Work out the finished part from the listing and answer in its coordinate system (mm). Face numbers are marked on the shaded views. A direction names the side the tool comes from. Coordinates: 2 decimals unless noted, no trailing zeros. Order: outer loops, then holes, each group sorted by start corner. A loop starts at its lowest first (then second) coordinate and runs counter-clockwise, first axis right, second up. Notation, with made-up numbers: M 45,-24.5 L 73,-24.5 A18 ccw 73,5.5 Z; hole C 17.25,10.5 d1. An arc over 180 degrees is marked long. Answer in a Markdown table with one row per item. Add a question column.
Item 1: The part is cut by section A-A (z = 4). Write down the section's boundary in (x, y), then the cut area to 3 significant figures.
Item 2: Which of the six approach directions +Z, -Z, +X, -X, +Y, -Y give full straight-line access (tool end or side, diameter ignored) to the marked faces 4, 5, 6 and 7?
Item 3: Consider line 1 (X direction, y = 8.25, z = -15); line 2 (Y direction, x = -2.5, z = -71); line 3 (Y direction, x = 17, z = -2). Determine where each line is inside the solid, lowest interval first. Write a range as from..to.
Item 4: The mould has two halves that part along Y. Classify the marked faces 1, 2 and 3: released by +Y, released by -Y, zero draft, split by the parting line, or undercut.
Item 5: The part is cut by section D-D (y = -28). Write down the section's boundary in (x, z), then the cut area to 3 significant figures.
Item 6: The part is cut by section C-C (y = 42). Write down the section's boundary in (x, z).
Item 7: Flat-ended cylindrical pins translate along their axes: pin 1 Ø8 at (x, y) = (-1, -16.5) entering from +Z; pin 2 Ø7 at (x, z) = (-9, 9) entering from +Y; pin 3 Ø17.5 at (y, z) = (-16, -99.5) entering from +X; pin 4 Ø10 at (x, z) = (13, -78) entering from +Y. Find the tip coordinate at first contact, or state that the pin passes through.
from build123d import *

# Parameters (mm, degrees)
SKETCH1_W                = 50
SKETCH1_H                = 140
BOSS_EXTRUDE1_DEPTH      = 10
SKETCH2_R                = 4.35
BOSS_EXTRUDE2_DEPTH      = 3
CIRPATTERN2_COUNT        = 8
SKETCH4_R                = 4.575
CUT_EXTRUDE3_DEPTH       = 3
SKETCH5_W                = 50
SKETCH5_H                = 10
BOSS_EXTRUDE3_DEPTH      = 70
SKETCH6_W                = 50
SKETCH6_H                = 50
CUT_EXTRUDE4_DEPTH       = 10
SKETCH7_R                = 1.75
CUT_EXTRUDE5_DEPTH       = 10
SKETCH8_W                = 4
SKETCH8_H                = 160
CUT_EXTRUDE6_DEPTH       = 10
CUT_EXTRUDE10_DEPTH      = 10
CUT_EXTRUDE9_DEPTH       = 10
SKETCH11_W               = 31.31699353
SKETCH11_H               = 105.183771494
BOSS_EXTRUDE4_DEPTH      = 40
FILLET1_R                = 20
FILLET2_R                = 20
SKETCH16_R               = 8
CUT_EXTRUDE15_DEPTH      = 10
CUT_EXTRUDE17_DEPTH      = 148.732867027
CUT_EXTRUDE17_DEPTH_BACK = 35
SKETCH18_W               = 31.31699353
SKETCH18_H               = 105.183771494
BOSS_EXTRUDE6_DEPTH      = 30
CUT_EXTRUDE20_DEPTH      = 164.171688721
CUT_EXTRUDE20_DEPTH_BACK = 30
SKETCH22_W               = 30.656149889
SKETCH22_H               = 104.820059864
BOSS_EXTRUDE7_DEPTH      = 5
SKETCH23_W               = 31.31699353
SKETCH23_H               = 20
CUT_EXTRUDE21_DEPTH      = 40
SKETCH24_W               = 30.656149889
SKETCH24_H               = 20
CUT_EXTRUDE22_DEPTH      = 35
SKETCH25_W               = 1.83885533
SKETCH25_H               = 1.068287382
CUT_EXTRUDE23_DEPTH      = 40
FILLET3_R                = 5
FILLET4_R                = 5


with BuildPart() as part:
    # Sketch1 → Boss-Extrude1 (new body)
    with BuildSketch(Plane(origin=(0, 0, 0), x_dir=(1, 0, 0), z_dir=(0, 1, 0))):
        Rectangle(SKETCH1_W, SKETCH1_H)
    extrude(amount=BOSS_EXTRUDE1_DEPTH)

    # Sketch2 → Boss-Extrude2 (add)
    with BuildSketch(Plane(origin=(0, 10, 0), x_dir=(1, 0, 0), z_dir=(0, 1, 0))):
        with Locations(Location((-14.25, 0, 0), (0, 0, 270))):
            Circle(SKETCH2_R)
    boss_extrude2 = extrude(amount=BOSS_EXTRUDE2_DEPTH)

    # CirPattern2: Boss-Extrude2 ×8 about axis
    cirpattern2_axis = Axis((0.122053198, 0, 0), (0, 1, 0))
    for i in range(1, CIRPATTERN2_COUNT):
        add(boss_extrude2.rotate(cirpattern2_axis, i * 360 / CIRPATTERN2_COUNT))

    # Sketch4 → Cut-Extrude3 (cut)
    with BuildSketch(Plane(origin=(0, 13, 0), x_dir=(1, 0, 0), z_dir=(0, 1, 0))):
        with Locations((-14.25, 0)):
            Circle(SKETCH4_R)
        with Locations((14.494106396, 0)):
            Circle(SKETCH4_R)
        with Locations((0.122053198, -14.372053198)):
            Circle(SKETCH4_R)
        with Locations((0.122053198, 14.372053198)):
            Circle(SKETCH4_R)
    extrude(amount=-CUT_EXTRUDE3_DEPTH, mode=Mode.SUBTRACT)

    # Sketch5 → Boss-Extrude3 (add)
    with BuildSketch(Plane(origin=(0, 0, -70), x_dir=(-1, 0, 0), z_dir=(0, 0, -1))):
        with Locations((0, 5)):
            Rectangle(SKETCH5_W, SKETCH5_H)
    extrude(amount=BOSS_EXTRUDE3_DEPTH)

    # Sketch6 → Cut-Extrude4 (cut)
    with BuildSketch(Plane(origin=(0, 10, 0), x_dir=(1, 0, 0), z_dir=(0, 1, 0))):
        with Locations((0, -45)):
            Rectangle(SKETCH6_W, SKETCH6_H)
    extrude(amount=-CUT_EXTRUDE4_DEPTH, mode=Mode.SUBTRACT)

    # Sketch7 → Cut-Extrude5 (cut)
    with BuildSketch(Plane(origin=(0, 10, 0), x_dir=(1, 0, 0), z_dir=(0, 1, 0))):
        with Locations(Location((15, 0, 0), (0, 0, 270))):
            Circle(SKETCH7_R)
        with Locations(Location((-15, 0, 0), (0, 0, 270))):
            Circle(SKETCH7_R)
        with Locations(Location((0, 15, 0), (0, 0, 270))):
            Circle(SKETCH7_R)
        with Locations(Location((0, -15, 0), (0, 0, 270))):
            Circle(SKETCH7_R)
    extrude(amount=-CUT_EXTRUDE5_DEPTH, mode=Mode.SUBTRACT)

    # Sketch8 → Cut-Extrude6 (cut)
    with BuildSketch(Plane(origin=(0, 10, 0), x_dir=(1, 0, 0), z_dir=(0, 1, 0))):
        with Locations((-23, 60)):
            Rectangle(SKETCH8_W, SKETCH8_H)
    extrude(amount=-CUT_EXTRUDE6_DEPTH, mode=Mode.SUBTRACT)

    # Sketch9 → Cut-Extrude10 (cut)
    with BuildSketch(Plane(origin=(0, 0, 0), x_dir=(-1, 0, 0), z_dir=(0, -1, 0))):
        Polygon((-10.051648387, 140), (-25, 61.50558626), (-25, 140), align=None)
    extrude(amount=-CUT_EXTRUDE10_DEPTH, mode=Mode.SUBTRACT)

    # Sketch10 → Cut-Extrude9 (cut)
    with BuildSketch(Plane(origin=(0, 0, 0), x_dir=(-1, 0, 0), z_dir=(0, -1, 0))):
        with BuildLine():
            Line((21, 34.816228506), (21, 140))
            ThreePointArc((21, 140), (-2.203275532, 87.408114253), (21, 34.816228506))
        make_face()
    extrude(amount=-CUT_EXTRUDE9_DEPTH, mode=Mode.SUBTRACT)

    # Sketch11 → Boss-Extrude4 (add)
    with BuildSketch(Plane(origin=(0, 10, 0), x_dir=(1, 0, 0), z_dir=(0, 1, 0))):
        with Locations((-5.606848378, 87.408114253)):
            Rectangle(SKETCH11_W, SKETCH11_H)
    extrude(amount=BOSS_EXTRUDE4_DEPTH)

    # Fillet1
    fillet1_edges = [part.edges().sort_by_distance(p)[0] for p in [
        (25, 5, 20),
    ]]
    fillet(fillet1_edges, radius=FILLET1_R)

    # Fillet2
    fillet2_edges = [part.edges().sort_by_distance(p)[0] for p in [
        (-21, 5, 20),
    ]]
    fillet(fillet2_edges, radius=FILLET2_R)

    # Sketch16 → Cut-Extrude15 (cut)
    with BuildSketch(Plane(origin=(0, 10, 0), x_dir=(1, 0, 0), z_dir=(0, 1, 0))):
        with Locations(Location((0, 0, 0), (0, 0, 270))):
            Circle(SKETCH16_R)
    extrude(amount=-CUT_EXTRUDE15_DEPTH, mode=Mode.SUBTRACT)

    # Sketch17 → Cut-Extrude17 (cut, two sides: drawn at the far end of the back side and taken through both)
    with BuildSketch(Plane(origin=(0, 10, 0), x_dir=(-1, 0, 0), z_dir=(0, -1, 0)).offset(-CUT_EXTRUDE17_DEPTH_BACK)):
        with BuildLine():
            Line((274.317595229, 371.200011147), (21, 140))
            ThreePointArc((21, 140), (-2.203275532, 87.408114253), (21, 34.816228506))
            Line((21, 34.816228506), (274.317595229, -196.383782641))
            Line((274.317595229, -196.383782641), (960.242515922, -196.383782641))
            Line((960.242515922, -196.383782641), (960.242515922, 371.200011147))
            Line((960.242515922, 371.200011147), (274.317595229, 371.200011147))
        make_face()
    extrude(amount=CUT_EXTRUDE17_DEPTH + CUT_EXTRUDE17_DEPTH_BACK, mode=Mode.SUBTRACT)

    # Sketch18 → Boss-Extrude6 (add)
    with BuildSketch(Plane(origin=(0, 0, 0), x_dir=(-1, 0, 0), z_dir=(0, -1, 0))):
        with Locations((5.606848378, 87.408114253)):
            Rectangle(SKETCH18_W, SKETCH18_H)
    extrude(amount=BOSS_EXTRUDE6_DEPTH)

    # Sketch21 → Cut-Extrude20 (cut, two sides: drawn at the far end of the back side and taken through both)
    with BuildSketch(Plane(origin=(0, -30, 0), x_dir=(-1, 0, 0), z_dir=(0, -1, 0)).offset(-CUT_EXTRUDE20_DEPTH_BACK)):
        with BuildLine():
            Line((268.426015736, 377.982607024), (21.265345143, 140))
            ThreePointArc((21.265345143, 140), (-1.103993451, 87.408114253), (21.265345143, 34.816228506))
            Line((21.265345143, 34.816228506), (268.426015736, -203.166378519))
            Line((268.426015736, -203.166378519), (954.644984679, -203.166378519))
            Line((954.644984679, -203.166378519), (954.644984679, 377.982607024))
            Line((954.644984679, 377.982607024), (268.426015736, 377.982607024))
        make_face()
    extrude(amount=CUT_EXTRUDE20_DEPTH + CUT_EXTRUDE20_DEPTH_BACK, mode=Mode.SUBTRACT)

    # Sketch22 → Boss-Extrude7 (add)
    with BuildSketch(Plane(origin=(0, -30, 0), x_dir=(-1, 0, 0), z_dir=(0, -1, 0))):
        with Locations((5.276426558, 87.589970068)):
            Rectangle(SKETCH22_W, SKETCH22_H)
    extrude(amount=BOSS_EXTRUDE7_DEPTH)

    # Sketch23 → Cut-Extrude21 (cut)
    with BuildSketch(Plane(origin=(0, 50, 0), x_dir=(1, 0, 0), z_dir=(0, 1, 0))):
        with Locations((-5.606848378, 44.816228506)):
            Rectangle(SKETCH23_W, SKETCH23_H)
    extrude(amount=-CUT_EXTRUDE21_DEPTH, mode=Mode.SUBTRACT)

    # Sketch24 → Cut-Extrude22 (cut)
    with BuildSketch(Plane(origin=(0, -35, 0), x_dir=(-1, 0, 0), z_dir=(0, -1, 0))):
        with Locations((5.276426558, 44.816228506)):
            Rectangle(SKETCH24_W, SKETCH24_H)
    extrude(amount=-CUT_EXTRUDE22_DEPTH, mode=Mode.SUBTRACT)

    # Sketch25 → Cut-Extrude23 (cut)
    with BuildSketch(Plane(origin=(0, -30, 0), x_dir=(-1, 0, 0), z_dir=(0, -1, 0))):
        with Locations((20.840871232, 35.107558697)):
            Rectangle(SKETCH25_W, SKETCH25_H)
    extrude(amount=-CUT_EXTRUDE23_DEPTH, mode=Mode.SUBTRACT)

    # Fillet3
    fillet3_edges = [part.edges().sort_by_distance(p)[0] for p in [
        (-21.265345143, 45, -97.408114253),
    ]]
    fillet(fillet3_edges, radius=FILLET3_R - 0.0001)  # a hair under: the kernel refuses the full size

    # Fillet4
    fillet4_edges = [part.edges().sort_by_distance(p)[0] for p in [
        (-20.604501502, -30, -97.085912401),
    ]]
    fillet(fillet4_edges, radius=FILLET4_R - 0.0001)  # a hair under: the kernel refuses the full size


solid = part.part
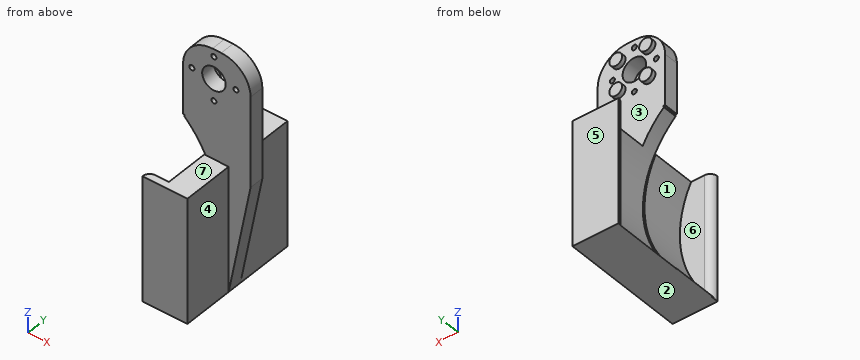
Reply:
| question | item | result |
|---|---|---|
| 1 | outline | M -20.6,0 L -6.93,0 L -6.93,10 L -20.6,10 Z; M 6.93,0 L 24.6,0 L 24.6,10 L 6.93,10 Z |
| 1 | area | 313 mm2 |
| 2 | face 4 | +Z, -Z, +X, -Y |
| 2 | face 5 | +Z, -Z, +X, -X, +Y |
| 2 | face 6 | -X |
| 2 | face 7 | +Z, +X, -X, -Y |
| 3 | line 1 | x = -21..-1.75, 1.75..25 |
| 3 | line 2 | y = -35..-30, 45..50 |
| 3 | line 3 | y = 0..10 |
| 4 | face 1 | undercut |
| 4 | face 2 | zero draft |
| 4 | face 3 | released by +Y |
| 5 | outline | M -21.27,-140 L 10.05,-140 L 10.05,-54.82 L -6.57,-54.82 A73.01 cw Z |
| 5 | area | 1,210 mm2 |
| 6 | outline | M -21,-140 L 10.05,-140 L 10.05,-54.82 L -5.69,-54.82 A71.2 cw Z |
| 7 | pin 1 | stops at z = -54.82 |
| 7 | pin 2 | stops at y = 13 |
| 7 | pin 3 | stops at x = 10.05 |
| 7 | pin 4 | stops at y = 50 |
